Print and shaded views of the part. All mm, measured from the part's lowest x, y and z. A direction names the side the tool comes from. Round coordinates to 2 decimals unless told otherwise and drop trailing zeros. Loops run counter-clockwise (first coordinate to the right, second up) from the corner with the lowest first, then second, coordinate; pieces in that order, holes last. Notation, with made-up numbers: (83, 68) - (118, 68) arc R24 ccw to (118, 104) - close; hole circle Ø1 at (39.5, 25.5). An arc over 180 degrees is marked (long way). Answer as a JSON object with one key per item and string values.
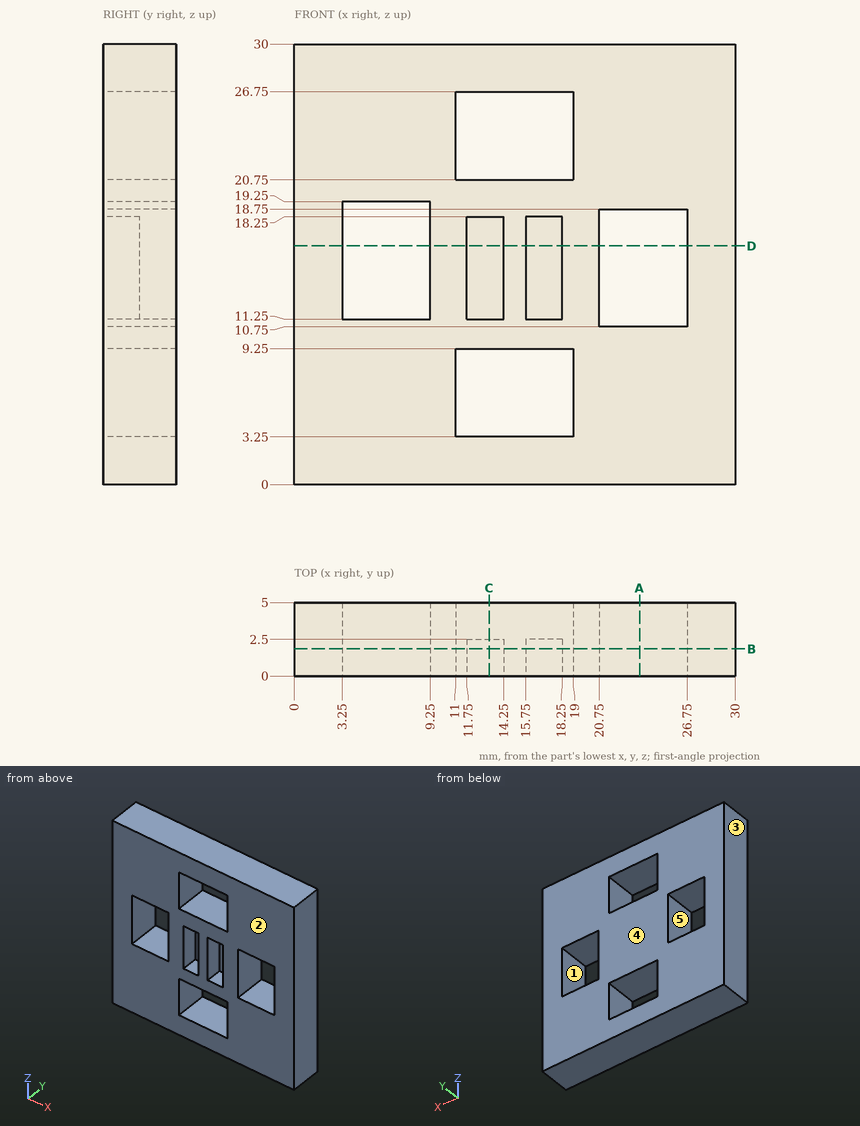
1) Tool access for the marked faces 4 and 5: list every direction of +Z, -Z, +X, -X, +Y, -Y with a clear straight run to the whole face (end or side of a thin tool).
Values follow:
{"face 4": "+Z, -Z, +X, -X, +Y", "face 5": "+Y, -Y"}
2) Slice it at A-A on x = 23.5. List the corners of the cut face in (y, z).
Values follow:
{"outline": "(0, 0) - (5, 0) - (5, 10.75) - (0, 10.75) - close; (0, 18.75) - (5, 18.75) - (5, 30) - (0, 30) - close"}
3) Two-plate mould, pull along X, no slides. Class the marked faces 1, 2 and 3: pulls with the +X half, pulls with the -X half, needs draft (parallel to the pull), parting line crosses it, or undercut.
Values follow:
{"face 1": "undercut", "face 2": "needs draft", "face 3": "pulls with the -X half"}
4) Drop a flat-ended pin along its axis: P1, Ø1.5, axis at y = 4.5, z = 16, coming from the -X side. Give the stop position or say it passes through.
Values follow:
{"P1": "x = 0"}
5) Slice it at D-D on z = 16.25. List the corners of the cut face in (x, y), then the cut area to 3 significant figures.
Values follow:
{"outline": "(0, 0) - (3.25, 0) - (3.25, 5) - (0, 5) - close; (9.25, 0) - (11.75, 0) - (11.75, 2.5) - (14.25, 2.5) - (14.25, 0) - (15.75, 0) - (15.75, 2.5) - (18.25, 2.5) - (18.25, 0) - (20.75, 0) - (20.75, 5) - (9.25, 5) - close; (26.75, 0) - (30, 0) - (30, 5) - (26.75, 5) - close", "area": "77.5 mm²"}
6) Slice it at C-C on x = 13.25. List the corners of the cut face in (y, z), then the cut area to 3 significant figures.
Values follow:
{"outline": "(0, 0) - (5, 0) - (5, 3.25) - (0, 3.25) - close; (0, 9.25) - (5, 9.25) - (5, 20.75) - (0, 20.75) - (0, 18.25) - (2.5, 18.25) - (2.5, 11.25) - (0, 11.25) - close; (0, 26.75) - (5, 26.75) - (5, 30) - (0, 30) - close", "area": "72.5 mm²"}
7) Probe probe 1 along Z at (x, y) = (12, 1.3); probe 2 along X at (y, z) = (2.8, 13.75). List the from-to ranges inside material, lowest first.
Values follow:
{"probe 1": "0 to 3.25, 9.25 to 11.25, 18.25 to 20.75, 26.75 to 30", "probe 2": "0 to 3.25, 9.25 to 20.75, 26.75 to 30"}
8) Slice it at B-B on y = 1.85. List the corners of the cut face in (x, z), then the cut area to 3 significant figures.
Values follow:
{"outline": "(0, 0) - (30, 0) - (30, 30) - (0, 30) - close; hole (3.25, 11.25) - (9.25, 11.25) - (9.25, 19.25) - (3.25, 19.25) - close; hole (11, 3.25) - (19, 3.25) - (19, 9.25) - (11, 9.25) - close; hole (11, 20.75) - (19, 20.75) - (19, 26.75) - (11, 26.75) - close; hole (11.75, 11.25) - (14.25, 11.25) - (14.25, 18.25) - (11.75, 18.25) - close; hole (15.75, 11.25) - (18.25, 11.25) - (18.25, 18.25) - (15.75, 18.25) - close; hole (20.75, 10.75) - (26.75, 10.75) - (26.75, 18.75) - (20.75, 18.75) - close", "area": "673 mm²"}
